```python
from build123d import *

# Parameters (mm, degrees)
F0_R     = 15.9004
F1_DEPTH = 7.239
F2_R     = 3.7973
F3_DEPTH = 14.479
F6_W     = 3.2282739412
F6_H     = 3.175


with BuildPart() as f1:
    # F0 (on Top) → F1 (new body, symmetric)
    with BuildSketch(Plane.XY):
        Circle(F0_R)
    extrude(amount=F1_DEPTH, both=True)

    # F2 (on face) → F3 (cut, through all)
    with BuildSketch(Plane.XY.offset(7.239)):
        Circle(F2_R)
    extrude(amount=-F3_DEPTH, mode=Mode.SUBTRACT)

    # F4 (on Right) → F5 (revolve, cut)
    with BuildSketch(Plane.YZ):
        Polygon((21.4757, -4.7117), (21.4757, 4.7117), (12.3317, 4.7117), (7.62, 0), (12.3317, -4.7117), align=None)
        Polygon((12.0194002201, 9.2803370403), (5.715, 9.2803370403), (5.715, 2.9428403359), align=None)
    revolve(axis=Axis((0, 0, 7.4247815646), (0, 0, 1)), mode=Mode.SUBTRACT)

    # F6 (on face) → F7 (join, up to the next surface of F1)
    with BuildSketch(Plane.XY.offset(7.239)):
        with Locations((0, 6.4679230563)):
            Rectangle(F6_W, F6_H)
    extrude(until=Until.NEXT, dir=(0, 0, -1))


solid = f1.part
```
The model under review builds one solid part; all positions refer to its coordinate system, in mm. A direction names the side the tool comes from. Round coordinates to 2 decimals unless told otherwise and drop trailing zeros. Write each loop counter-clockwise with the first axis right and the second up, starting at its lowest first coordinate (ties: lowest second). Pieces come first, ordered by that corner, then holes. Notation, with made-up numbers: (29.5, 24) - (72.5, 24) arc R32 ccw to (72.5, 61) - close; hole circle Ø10 at (22, 50). An arc over 180 degrees is marked (long way). Use one line per item in the form item = value.
Q1. Consider section B-B (x = 0). State the section outline as (y, z) points (3 decimals), and give its area (3 significant figures).
Answer key:
outline = (-15.9, -7.239) - (-3.797, -7.239) - (-3.797, 7.239) - (-5.715, 7.239) - (-5.715, 2.943) - (-9.989, 7.239) - (-15.9, 7.239) - (-15.9, 4.712) - (-12.332, 4.712) - (-7.62, 0) - (-12.332, -4.712) - (-15.9, -4.712) - close; (3.797, -7.239) - (15.9, -7.239) - (15.9, -4.712) - (12.332, -4.712) - (7.62, 0) - (12.332, 4.712) - (15.9, 4.712) - (15.9, 7.239) - (9.989, 7.239) - (8.055, 5.296) - (8.055, 7.239) - (3.797, 7.239) - close
area = 228 mm2
Q2. Draft analysis for pull direction Y (two halves, no side actions). For faces 4 (the flat face through (0, 8.055, 6)), 5 (the conical face through (-2.358, 7.486, 0.229)), 6 (the flat face through (-3, 3, 7.239)), 7 (the conical face through (5.84, -1.3, 3.21)), state which applies: +Y half, -Y half, draft (parallel to the pull), parting line (faces both ways), or undercut.
Answer key:
face_4 = undercut
face_5 = parting line
face_6 = draft
face_7 = undercut
Q3. Tool access review of faces 1 (the flat face through (-1.614, 6, 6)), 2 (the cylindrical face through (-3.45, -15.52, 5.99)), 3 (the flat face through (12, -5, -4.712)): name each direction out of +Z, -Z, +X, -X, +Y, -Y from which nothing blocks a thin tool from reaching the whole face with its end or side.
Answer key:
face_1 = +Z
face_2 = +Z, -Z
face_3 = none
Q4. Consider section A-A (y = 0). State the section outline as (x, z) points (3 decimals), and give its area (3 significant figures).
Answer key:
outline = (-15.9, -7.239) - (-3.797, -7.239) - (-3.797, 7.239) - (-5.715, 7.239) - (-5.715, 2.943) - (-9.989, 7.239) - (-15.9, 7.239) - (-15.9, 4.712) - (-12.332, 4.712) - (-7.62, 0) - (-12.332, -4.712) - (-15.9, -4.712) - close; (3.797, -7.239) - (15.9, -7.239) - (15.9, -4.712) - (12.332, -4.712) - (7.62, 0) - (12.332, 4.712) - (15.9, 4.712) - (15.9, 7.239) - (9.989, 7.239) - (5.715, 2.943) - (5.715, 7.239) - (3.797, 7.239) - close
area = 220 mm2
Q5. Consider section D-D (y = 14.5). State the section outline as (x, z) points.
Answer key:
outline = (-6.52, -7.24) - (6.52, -7.24) - (6.52, -4.71) - (-6.52, -4.71) - close; (-6.52, 4.71) - (6.52, 4.71) - (6.52, 7.24) - (-6.52, 7.24) - close
Q6. For line 1 (Z direction, x = -3, y = -14.5); line 2 (Y direction, x = 1, z = 5.25); line 3 (Y direction, x = -5, z = 4.5), list the stretches that pass through material, from the lowest coordinate up. Write a range as [from, to].
Answer key:
line_1 = [-7.24, -4.71], [4.71, 7.24]
line_2 = [-15.87, -7.95], [-5.63, -3.66], [3.66, 15.87]
line_3 = [-11.04, -5.27], [-2.77, 2.77], [5.27, 11.04]
Q7. Consider section C-C (z = -2.75). State the section outline as (x, y) points, and give its area (3 significant figures).
Answer key:
outline = circle Ø20.74 at (0, 0); hole circle Ø7.59 at (0, 0)
area = 293 mm2
Q8. Insertion check: pin 1 Ø5 at (x, z) = (3.5, -1) entering from +Y; pin 2 Ø8 at (y, z) = (-7.5, -4) entering from -X; pin 3 Ø1 at (x, z) = (9.5, -3.5) entering from -Y. Each pin has a flat end and moves straight along its axis. Give the tip position at first contact, or say it passes through.
Answer key:
pin_1 = 10.66
pin_2 = -15.5
pin_3 = -6.93
